```python
from build123d import *

# Parameters (mm, degrees)
SKETCH1_W           = 40.64
SKETCH1_H           = 40.64
BOSS_EXTRUDE1_DEPTH = 59.182
SKETCH2_W           = 40.64
SKETCH2_H           = 40.64
BOSS_EXTRUDE2_DEPTH = 17.78
SHELL1_START        = -36.762774376
SHELL1_OUTLINE_W    = 54.102
SHELL1_OUTLINE_H    = 35.56
SHELL1_DEPTH        = 35.56
SHELL1_START_2      = -1.202774376
SHELL1_2_OUTLINE_W  = 35.56
SHELL1_2_OUTLINE_H  = 35.56
SHELL1_2_DEPTH      = 17.78


# Read off the part's stored shape, not the designer's step: Shell1
with BuildPart() as part:
    # Sketch1 → Boss-Extrude1 (new body)
    with BuildSketch(Plane(origin=(0, 0, 0), x_dir=(1, 0, 0), z_dir=(0, 1, 0))):
        with Locations((-18.982774376, 6.236831683)):
            Rectangle(SKETCH1_W, SKETCH1_H)
    extrude(amount=BOSS_EXTRUDE1_DEPTH)

    # Sketch2 → Boss-Extrude2 (add)
    with BuildSketch(Plane(origin=(1.337225624, 0, 0), x_dir=(0, 0, -1), z_dir=(1, 0, 0))):
        with Locations((6.236831683, 20.32)):
            Rectangle(SKETCH2_W, SKETCH2_H)
    extrude(amount=BOSS_EXTRUDE2_DEPTH)

    # Shell1 outline → Shell1 (cut)
    with BuildSketch(Plane.YZ.offset(SHELL1_START)):
        with Locations((29.591, -6.236831683)):
            Rectangle(SHELL1_OUTLINE_W, SHELL1_OUTLINE_H)
    extrude(amount=SHELL1_DEPTH, mode=Mode.SUBTRACT)

    # Shell1 2 outline → Shell1 2 (cut)
    with BuildSketch(Plane.YZ.offset(SHELL1_START_2)):
        with Locations((20.32, -6.236831683)):
            Rectangle(SHELL1_2_OUTLINE_W, SHELL1_2_OUTLINE_H)
    extrude(amount=SHELL1_2_DEPTH, mode=Mode.SUBTRACT)


solid = part.part
```
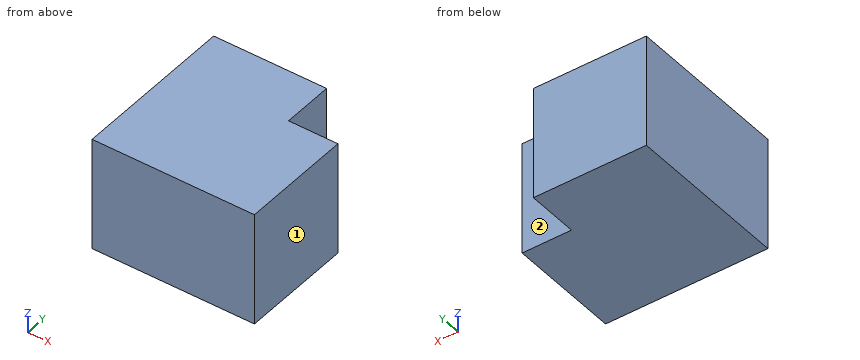
Input: part model. Units: mm. Frame: model coordinates. Face numbers are marked on the shaded views. A direction names the side the tool comes from. Give positions to 0.01 mm unless a question says otherwise; leave off trailing zeros. Order: outer loops, then holes, each group sorted by start corner. A loop starts at its lowest first (then second) coordinate and runs counter-clockwise, first axis right, second up. Notation, with made-up numbers: M 63.5,14 L 108.5,14 A19 ccw 108.5,51 Z; hole C 38.25,-24 d10. An arc over 180 degrees is marked long. One line per question, with ' | ' between items.
1) Section B-B on y = 24.5. Output: boundary loops of the cut face in (x, z), and give its area (3 significant figures).
Filled in:
outline: M -39.3,-26.56 L 19.12,-26.56 L 19.12,14.08 L -39.3,14.08 Z; hole M -36.76,-24.02 L 16.58,-24.02 L 16.58,11.54 L -36.76,11.54 Z | area: 477 mm2
2) Contact query for a flat-ended pin moving along its axis: P1, Ø5.5, axis at y = 51, z = -1, coming from the +X side. Output: stop coordinate, or through.
Filled in:
P1: stops at x = 1.34
3) Section C-C on z = 5. Output: boundary loops of the cut face in (x, y).
Filled in:
outline: M -39.3,0 L 19.12,0 L 19.12,40.64 L 1.34,40.64 L 1.34,59.18 L -39.3,59.18 Z; hole M -36.76,2.54 L 16.58,2.54 L 16.58,38.1 L -1.2,38.1 L -1.2,56.64 L -36.76,56.64 Z
4) Access query for the marked faces 1 and 2. Directions: +Z, -Z, +X, -X, +Y, -Y. A direction counts if a zero-diameter tool reaches every point of the face in a straight line with its end or side. Return the directions, or none.
Filled in:
face 1: +Z, -Z, +X, +Y, -Y | face 2: +Z, -Z, +X, +Y
5) Section A-A on x = 3. Output: boundary loops of the cut face in (y, z).
Filled in:
outline: M 0,-26.56 L 40.64,-26.56 L 40.64,14.08 L 0,14.08 Z; hole M 2.54,-24.02 L 38.1,-24.02 L 38.1,11.54 L 2.54,11.54 Z
6) Ray query, L1, parallel to Z at x = -32, y = 6.5; L2, parallel to Y at x = -14, z = -19; L3, parallel to Y at x = 8.5, z = 2. Return the intervals inside material, ascending.
Filled in:
L1: z = -26.56 to -24.02, 11.54 to 14.08 | L2: y = 0 to 2.54, 56.64 to 59.18 | L3: y = 0 to 2.54, 38.1 to 40.64
